Part model, mm, in its own coordinate system. Face numbers are marked on the shaded views. Give positions to 0.01 mm unless a question says otherwise; leave off trailing zeros. Write each loop counter-clockwise with the first axis right and the second up, starting at its lowest first coordinate (ties: lowest second). Pieces come first, ordered by that corner, then holes. Notation, with made-up numbers: M -16.5,8 L 6.5,8 A33 ccw 6.5,37 Z; hole C 25.25,69.25 d5. An arc over 180 degrees is marked long. Answer as CSV lines item,"result". Start each with the question number.
1) Mould opens along X. For the marked faces 1 and 2 say: pulls with the +X half, pulls with the -X half, needs draft (parallel to the pull), parting line crosses it, or undercut.
2) Wall check: line 1 along X through (y, z) = (-1.9, 38.06); line 2 along Z through (x, y) = (7.5, 8); line 3 along Y through (x, z) = (13, 22.5). Give the ranges that are in metal, low to high. Write a range as from..to.
3) Pin check, flat tips, straight feed: pin 1 Ø6 at (x, y) = (12.5, 23.5) entering from +Z; pin 2 Ø2.5 at (y, z) = (-2, 12) entering from -X; pin 3 Ø0.8 at (x, y) = (-23, 11) entering from +Z; pin 4 Ø2.5 at (y, z) = (35.5, 2) entering from -X. Stop position of each tip, or through.
4) Slice it at A-A, the plane z = 22.56. Give the cut face in (x, y).
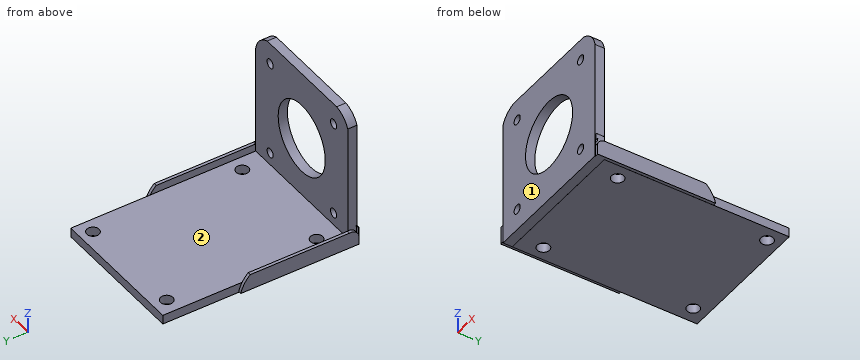
```python
from build123d import *

# Parameters (mm, degrees)
SKETCH_W        = 45
SKETCH_H        = 45
PAD_DEPTH       = 3
SKETCH007_W     = 45
SKETCH007_H     = 3
PAD001_DEPTH    = 60
POCKET_DEPTH    = 2.5
SKETCH004_R     = 11.5
SKETCH004_R_2   = 1.5
POCKET001_DEPTH = 3
SKETCH005_R     = 2
POCKET002_DEPTH = 5
SKETCH008_W     = 5.466466
SKETCH008_H     = 38.267721
PAD002_DEPTH    = 1
POCKET003_DEPTH = 1
SKETCH010_W     = 5.830426
SKETCH010_H     = 38.5055
PAD003_DEPTH    = 1
POCKET004_DEPTH = 1


with BuildPart() as part:
    # Sketch → Pad (new body)
    with BuildSketch(Plane.XZ):
        with Locations((0.043154, 22.5)):
            Rectangle(SKETCH_W, SKETCH_H)
    extrude(amount=PAD_DEPTH)

    # Sketch007 (on Face5 of Pad) → Pad001 (join)
    with BuildSketch(Plane(origin=(0, 0, 0), x_dir=(1, 0, 0), z_dir=(0, 1, 0))):
        with Locations((0.036956, -1.493426)):
            Rectangle(SKETCH007_W, SKETCH007_H)
    extrude(amount=PAD001_DEPTH)

    # Sketch003 → Pocket (cut, symmetric)
    with BuildSketch(Plane.XZ.offset(2)):
        with BuildLine():
            ThreePointArc((-16.103364, 45.081264), (-21.082356, 42.909937), (-23.129993, 37.878814))
            Line((-23.129993, 37.878814), (-23.129993, 45.081264))
            Line((-16.103364, 45.081264), (-23.129993, 45.081264))
        make_face()
        with BuildLine():
            ThreePointArc((22.687422, 37.148395), (20.279616, 42.961353), (14.466658, 45.369159))
            Line((14.466658, 45.369159), (22.687422, 45.369159))
            Line((22.687422, 37.148395), (22.687422, 45.369159))
        make_face()
    extrude(amount=POCKET_DEPTH, both=True, mode=Mode.SUBTRACT)

    # Sketch004 → Pocket001 (cut, symmetric)
    with BuildSketch(Plane.XZ.offset(2)):
        with Locations((0.049257, 22.56)):
            Circle(SKETCH004_R)
        with Locations((15.472322, 7.06)):
            Circle(SKETCH004_R_2)
        with Locations((-15.527678, 38.06)):
            Circle(SKETCH004_R_2)
        with Locations((15.472322, 38.06)):
            Circle(SKETCH004_R_2)
        with Locations((-15.527678, 7.06)):
            Circle(SKETCH004_R_2)
    extrude(amount=POCKET001_DEPTH, both=True, mode=Mode.SUBTRACT)

    # Sketch005 → Pocket002 (cut)
    with BuildSketch(Plane(origin=(0, 0, 3), x_dir=(-1, 0, 0), z_dir=(0, 0, 1))):
        with Locations((-17.816827, -7.458325)):
            Circle(SKETCH005_R)
        with Locations((18.098759, -7.214429)):
            Circle(SKETCH005_R)
        with Locations((-17.948954, -55.841232)):
            Circle(SKETCH005_R)
        with Locations((17.504663, -55.428982)):
            Circle(SKETCH005_R)
    extrude(amount=-POCKET002_DEPTH, mode=Mode.SUBTRACT)

    # Sketch008 (on Face11 of Pocket002) → Pad002 (join)
    with BuildSketch(Plane(origin=(22.536956, 0, 0), x_dir=(0, 0, 1), z_dir=(1, 0, 0))):
        with Locations((2.733233, -16.310083)):
            Rectangle(SKETCH008_W, SKETCH008_H)
    extrude(amount=PAD002_DEPTH)

    # Sketch009 (on Face27 of Pad002) → Pocket003 (cut)
    with BuildSketch(Plane(origin=(23.536956, 0, 0), x_dir=(0, 0, 1), z_dir=(1, 0, 0))):
        with BuildLine():
            ThreePointArc((5.454798, -0.127493), (5.024588, 1.810299), (3.367288, 2.902761))
            Line((3.367288, 2.902761), (7.963681, 2.626362))
            Line((7.963681, 2.626362), (7.963681, -32.524605))
            Line((7.963681, -32.524605), (6.482224, -36.026234))
            Line((6.482224, -36.026234), (0, -35.465638))
            ThreePointArc((0, -35.465638), (2.96164, -34.285148), (5.454798, -32.297931))
            Line((5.454798, -0.127493), (5.454798, -32.297931))
        make_face()
    extrude(amount=-POCKET003_DEPTH, mode=Mode.SUBTRACT)

    # Sketch010 (on Face2 of Pocket003) → Pad003 (join)
    with BuildSketch(Plane(origin=(-22.463044, 0, 0), x_dir=(0, 0, -1), z_dir=(-1, 0, 0))):
        with Locations((-3.174851, -16.191193)):
            Rectangle(SKETCH010_W, SKETCH010_H)
    extrude(amount=PAD003_DEPTH)

    # Sketch011 (on Face27 of Pad003) → Pocket004 (cut)
    with BuildSketch(Plane(origin=(-23.463044, 0, 0), x_dir=(0, 0, -1), z_dir=(-1, 0, 0))):
        with BuildLine():
            ThreePointArc((-3.367288, 2.902761), (-5.024589, 1.810299), (-5.454799, -0.127493))
            Line((-5.454799, -0.127493), (-5.454799, -32.297931))
            ThreePointArc((-5.454799, -32.297931), (-2.961641, -34.285149), (0, -35.465639))
            Line((-6.482224, -36.026234), (0, -35.465639))
            Line((-7.963681, -32.524605), (-6.482224, -36.026234))
            Line((-7.963681, 2.626362), (-7.963681, -32.524605))
            Line((-3.367288, 2.902761), (-7.963681, 2.626362))
        make_face()
    extrude(amount=-POCKET004_DEPTH, mode=Mode.SUBTRACT)


solid = part.part
```
Found:
1,face 1,"needs draft"
1,face 2,"undercut"
2,line 1,"-22.46..-17.03, -14.03..13.97, 16.97..22.54"
2,line 2,"-0.01..2.99"
2,line 3,"-3..0"
3,pin 1,"z = 2.99"
3,pin 2,"x = -22.46"
3,pin 3,"z = 5.45"
3,pin 4,"x = -23.46"
4,outline,"M -22.46,-3 L -11.45,-3 L -11.45,0 L -22.46,0 Z; M 11.55,-3 L 22.54,-3 L 22.54,0 L 11.55,0 Z"
